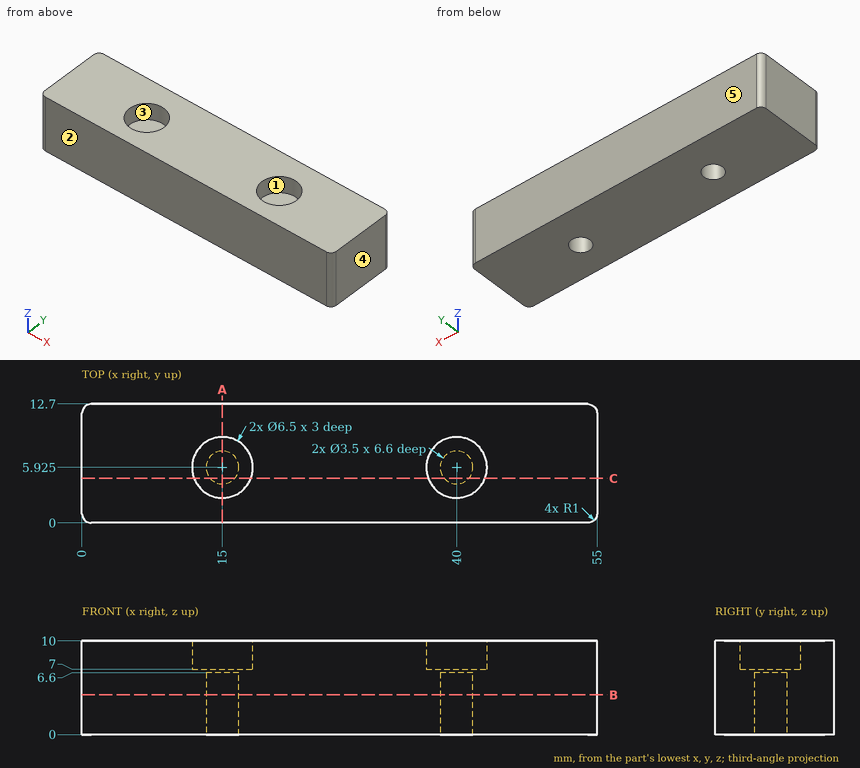
Source: three-view drawing plus pictorial views. Frame: mm from the lowest corner of the part. A direction names the side the tool comes from. Round coordinates to 2 decimals unless told otherwise and drop trailing zeros. Loops run counter-clockwise (first coordinate to the right, second up) from the corner with the lowest first, then second, coordinate; pieces in that order, holes last.
Q1. Section C-C on y = 4.75. Return loops of the section in (x, z).
Q2. Pin query (flat end, axial travel): P1, Ø5.5, axis at x = 15, y = 5.925, coming from the -Z side; P2, Ø1, axis at x = 40.5, y = 6.5, coming from the -Z side; P3, Ø5.5, axis at x = 40, y = 5.925, coming from the +Z side. Return the tip coordinate at first contact, or that it passes through.
Q3. Material intervals for L1, parallel to Y at x = 15, z = 8.2 (3 decimals); L2, parallel to X at y = 3.75, z = 9.5; L3, parallel to X at y = 5, z = 3.25, sorted ascending.
Q4. Pull-direction query (Y, two-part tool) for the marked faces 3, 4 and 5; classes: released by +Y, released by -Y, zero draft, split by the parting line, or undercut.
Q5. Section B-B on z = 4.25. Return loops of the section in (x, y) (3 decimals), plus the area to 3 significant figures.
Q6. Access query for the marked faces 1 and 2. Directions: +Z, -Z, +X, -X, +Y, -Y. A direction counts if a zero-diameter tool reaches every point of the face in a straight line with its end or side. Return the directions, or none.
Q7. Section A-A on x = 15. Return loops of the section in (y, z) (3 decimals), plus the area to 3 significant figures.
Evaluation:
1. outline: (0, 0) - (13.7, 0) - (13.7, 6.6) - (16.3, 6.6) - (16.3, 0) - (38.7, 0) - (38.7, 6.6) - (41.3, 6.6) - (41.3, 0) - (55, 0) - (55, 10) - (43.03, 10) - (43.03, 7) - (36.97, 7) - (36.97, 10) - (18.03, 10) - (18.03, 7) - (11.97, 7) - (11.97, 10) - (0, 10) - close
2. P1: stops at z = 0
2. P2: stops at z = 6.6
2. P3: stops at z = 7
3. L1: y = 0 to 2.675, 9.175 to 12.7
3. L2: x = 0 to 12.59, 17.41 to 37.59, 42.41 to 55
3. L3: x = 0 to 13.51, 16.49 to 38.51, 41.49 to 55
4. face 3: undercut
4. face 4: zero draft
4. face 5: released by +Y
5. outline: (0, 1) arc R1 ccw to (1, 0) - (54, 0) arc R1 ccw to (55, 1) - (55, 11.7) arc R1 ccw to (54, 12.7) - (1, 12.7) arc R1 ccw to (0, 11.7) - close; hole circle Ø3.5 at (15, 5.925); hole circle Ø3.5 at (40, 5.925)
5. area: 678 mm2
6. face 1: +Z
6. face 2: +Z, -Z, +X, -X, -Y
7. outline: (0, 0) - (4.175, 0) - (4.175, 6.6) - (7.675, 6.6) - (7.675, 0) - (12.7, 0) - (12.7, 10) - (9.175, 10) - (9.175, 7) - (2.675, 7) - (2.675, 10) - (0, 10) - close
7. area: 84.4 mm2
